from build123d import *

# Parameters (mm, degrees)
BOSS_EXTRU_1_DEPTH                              = 6
CHAMBRAGE_POUR_VIS_T_TE_CYLINDRIQUE_D           = 2.5
CHAMBRAGE_POUR_VIS_T_TE_CYLINDRIQUE_CBORE_D     = 4.5
CHAMBRAGE_POUR_VIS_T_TE_CYLINDRIQUE_CBORE_DEPTH = 4.5
CONG_1_R                                        = 0.5
ESQUISSE6_R                                     = 1.6
ENL_V_MAT_EXTRU_1_DEPTH                         = 17.673332037
ESQUISSE7_W                                     = 6
ESQUISSE7_H                                     = 2.25
ENL_V_MAT_EXTRU_2_DEPTH                         = 17.673332001


with BuildPart() as part:
    # Esquisse1 → Boss.-Extru.1 (new body)
    with BuildSketch(Plane(origin=(0, 0, 0), x_dir=(1, 0, 0), z_dir=(0, 1, 0))):
        with BuildLine():
            Line((4.582575695, 10), (-4.582575695, 10))
            ThreePointArc((-4.582575695, 10), (0, -11), (4.582575695, 10))
        make_face()
        with BuildLine():
            Line((-3.2, 0), (-3.2, 2.9))
            Line((-3.2, 2.9), (3.2, 2.9))
            Line((3.2, 2.9), (3.2, 0))
            ThreePointArc((3.2, 0), (0, -3.2), (-3.2, 0))
        make_face(mode=Mode.SUBTRACT)
    extrude(amount=BOSS_EXTRU_1_DEPTH)

    # Chambrage pour vis à tête cylindrique à 6 pans creux (ou vis CHC) M21 (through all)
    with Locations(Plane(origin=(0, 6, 0), x_dir=(1, 0, 0), z_dir=(0, 1, 0))):
        with Locations((5.656854249, 5.656854249), (5.656854249, -5.656854249), (-5.656854249, -5.656854249), (-5.656854249, 5.656854249), (0, 0)):
            CounterBoreHole(CHAMBRAGE_POUR_VIS_T_TE_CYLINDRIQUE_D / 2, CHAMBRAGE_POUR_VIS_T_TE_CYLINDRIQUE_CBORE_D / 2, CHAMBRAGE_POUR_VIS_T_TE_CYLINDRIQUE_CBORE_DEPTH)

    # Congé1
    cong_1_edges = [part.edges().sort_by_distance(p)[0] for p in [
        (0, 6, 3.2),
        (3.2, 6, -1.45),
        (0, 6, -2.9),
        (-3.2, 6, -1.45),
    ]]
    fillet(cong_1_edges, radius=CONG_1_R)

    # Esquisse6 → Enlèv. mat.-Extru.1 (cut, through all)
    with BuildSketch(Plane.XY):
        with Locations((0, 3.5)):
            Circle(ESQUISSE6_R)
    extrude(amount=-ENL_V_MAT_EXTRU_1_DEPTH, mode=Mode.SUBTRACT)

    # Esquisse7 → Enlèv. mat.-Extru.2 (cut, through all)
    with BuildSketch(Plane(origin=(0, 6, 0), x_dir=(1, 0, 0), z_dir=(0, 1, 0))):
        with Locations((0, 5.025)):
            Rectangle(ESQUISSE7_W, ESQUISSE7_H)
    extrude(amount=-ENL_V_MAT_EXTRU_2_DEPTH, mode=Mode.SUBTRACT)


solid = part.part
Input: part model. Units: mm. Frame: model coordinates. A direction names the side the tool comes from. Round coordinates to 2 decimals unless told otherwise and drop trailing zeros. Order: outer loops, then holes, each group sorted by start corner. A loop starts at its lowest first (then second) coordinate and runs counter-clockwise, first axis right, second up. Notation, with made-up numbers: (9.5, 16.25) - (28.5, 16.25) arc R20 ccw to (28.5, 21.25) - close; hole circle Ø8 at (27.25, 69). An arc over 180 degrees is marked (long way). Answer as a JSON object with one key per item and string values. Group by question number.
(1) Reachability of faces 5 (the face through (-6.145, 3.782, 7.853)), 6 (the face through (1, 2, -10)), 7 (the face through (3, 3, -5)), 8 (the face through (1.526, 3.981, -8.048)) from +Z, -Z, +X, -X, +Y, -Y: full face, straight path, thin tool, end or side. Return the list, or none.
(2) Draft query along X for faces 1 (the face through (2, 0, 3)), 2 (the face through (4.465, 0.739, 5.281)), 3 (the face through (0, 1.7, -3.9)), 4 (the face through (0, 3, 11)). Return one class per face: released by +X, released by -X, zero draft, split by the parting line, or undercut.
(3) Cut plane B-B (y = 3.5). Return loops of the section in (x, z), then the cut area to 3 significant figures.
(4) Cut plane A-A (x = 0). Return loops of the section in (y, z), then the cut area to 3 significant figures.
(5) Pin query (flat end, axial travel): P1, Ø4, axis at x = -0.5, z = -5, coming from the -Y side; P2, Ø1.3, axis at x = -6, z = -5, coming from the +Y side; P3, Ø3, axis at x = 0, y = 3.5, coming from the -Z side; P4, Ø3, axis at y = 2.5, z = -2.5, coming from the -X side. Return the tip coordinate at first contact, or that it passes through.
(6) Material intervals for probe 1 along Z at (x, y) = (-1.75, 2.5); probe 2 along Z at (x, y) = (3.75, 4.25); probe 3 along Y at (x, z) = (0, -6.85), sorted ascending. Write a range as from..to.
(7) Cut plane C-C (x = -5.5). Return loops of the section in (y, z).
(8) Cut plane D-D (y = 1). Return loops of the section in (x, z).
Here are the results:
{
 "1": {"face 5": "+Y", "face 6": "-Z, +X, -X, +Y, -Y", "face 7": "+Y, -Y", "face 8": "-Z"},
 "2": {"face 1": "zero draft", "face 2": "undercut", "face 3": "undercut", "face 4": "split by the parting line"},
 "3": {"outline": "(-4.58, -10) - (-1.6, -10) - (-1.6, -6.15) - (-3, -6.15) - (-3, -3.9) - (-1.6, -3.9) - (-1.6, -2.9) - (-3.2, -2.9) - (-3.2, 0) arc R3.2 cw to (3.2, 0) - (3.2, -2.9) - (1.6, -2.9) - (1.6, -3.9) - (3, -3.9) - (3, -6.15) - (1.6, -6.15) - (1.6, -10) - (4.58, -10) arc R11 ccw (long way) to start; hole circle Ø4.5 at (-5.66, -5.66); hole circle Ø4.5 at (-5.66, 5.66); hole circle Ø4.5 at (5.66, -5.66); hole circle Ø4.5 at (5.66, 5.66)", "area": "247 mm^2"},
 "4": {"outline": "(0, -10) - (1.9, -10) - (1.9, -6.15) - (0, -6.15) - close; (0, -3.9) - (1.9, -3.9) - (1.9, -2.9) - (0, -2.9) - close; (0, 3.2) - (5.5, 3.2) arc R0.5 ccw to (6, 3.7) - (6, 11) - (0, 11) - close; (5.1, -10) - (6, -10) - (6, -6.15) - (5.1, -6.15) - close; (5.1, -3.9) - (6, -3.9) - (6, -3.4) arc R0.5 ccw to (5.5, -2.9) - (5.1, -2.9) - close", "area": "60.3 mm^2"},
 "5": {"P1": "stops at y = 0", "P2": "stops at y = 1.5", "P3": "stops at z = 2.83", "P4": "stops at x = -10.95"},
 "6": {"probe 1": "z = -10..-6.15, -3.9..-2.9, 2.68..10.86", "probe 2": "z = -10..-6.85, -4.46..4.46, 6.85..10.34", "probe 3": "y = 0..1.9, 5.1..6"},
 "7": {"outline": "(0, -9.53) - (6, -9.53) - (6, -7.9) - (1.5, -7.9) - (1.5, -6.9) - (0, -6.9) - close; (0, -4.42) - (1.5, -4.42) - (1.5, -3.41) - (6, -3.41) - (6, 3.41) - (1.5, 3.41) - (1.5, 4.42) - (0, 4.42) - close; (0, 6.9) - (1.5, 6.9) - (1.5, 7.9) - (6, 7.9) - (6, 9.53) - (0, 9.53) - close"},
 "8": {"outline": "(-4.58, -10) - (4.58, -10) arc R11 ccw (long way) to start; hole circle Ø2.5 at (-5.66, -5.66); hole circle Ø2.5 at (-5.66, 5.66); hole (-3.2, -2.9) - (3.2, -2.9) - (3.2, 0) arc R3.2 ccw to (-3.2, 0) - close; hole (-3, -6.15) - (3, -6.15) - (3, -3.9) - (-3, -3.9) - close; hole circle Ø2.5 at (5.66, -5.66); hole circle Ø2.5 at (5.66, 5.66)"}
}
